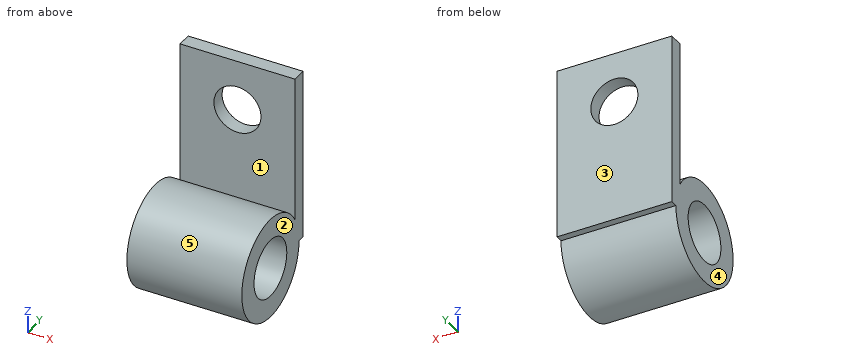
from build123d import *

# Parameters (mm, degrees)
LOOP_SKETCH_R       = 5.575
LOOP_DEPTH          = 6.35
TAB_SKETCH_W        = 18.94
TAB_SKETCH_H        = 1.6
TAB_DEPTH           = 6.35
TUBE_HOLE_SKETCH_R  = 3.195
TUBE_HOLE_DEPTH     = 7.35
MOUNT_HOLE_SKETCH_R = 2.6
MOUNT_HOLE_DEPTH    = 20


with BuildPart() as part:
    # Loop Sketch → Loop (new, symmetric)
    with BuildSketch(Plane(origin=(0, 0, 0), x_dir=(0, 0, -1), z_dir=(1, 0, 0))):
        Circle(LOOP_SKETCH_R)
    extrude(amount=LOOP_DEPTH, both=True)

    # Tab Sketch → Tab (add, symmetric)
    with BuildSketch(Plane(origin=(0, 0, 0), x_dir=(0, 0, -1), z_dir=(1, 0, 0))):
        with Locations((-9.47, 5.575)):
            Rectangle(TAB_SKETCH_W, TAB_SKETCH_H)
    extrude(amount=TAB_DEPTH, both=True)

    # Tube Hole Sketch → Tube Hole (cut, symmetric)
    with BuildSketch(Plane(origin=(0, 0, 0), x_dir=(0, 0, -1), z_dir=(1, 0, 0))):
        Circle(TUBE_HOLE_SKETCH_R)
    extrude(amount=TUBE_HOLE_DEPTH, both=True, mode=Mode.SUBTRACT)

    # Mount Hole Sketch → Mount Hole (cut, symmetric)
    with BuildSketch(Plane(origin=(0, 0, 0), x_dir=(1, 0, 0), z_dir=(0, 1, 0))):
        with Locations(Location((0, -13.44, 0), (0, 0, 270))):
            Circle(MOUNT_HOLE_SKETCH_R)
    extrude(amount=MOUNT_HOLE_DEPTH, both=True, mode=Mode.SUBTRACT)


solid = part.part
Design review of the part built by this model. Coordinates are the model's own, in mm. Face numbers are marked on the shaded views. A direction names the side the tool comes from. Give positions to 0.01 mm unless a question says otherwise; leave off trailing zeros. Order: outer loops, then holes, each group sorted by start corner. A loop starts at its lowest first (then second) coordinate and runs counter-clockwise, first axis right, second up. Notation, with made-up numbers: (-15.75, -39) - (8.25, -39) arc R12 ccw to (8.25, -21) - close; hole circle Ø10 at (-32, 40.5). An arc over 180 degrees is marked (long way). Use CSV: the item, a comma, the result in double quotes. Start each with the question number.
Q1. Take a section at B-B (y = 0). State the section outline as (x, z) points (3 decimals).
Q2. Draft analysis for pull direction Y (two halves, no side actions). For the marked faces 3, 4 and 5, state which applies: pulls with the +Y half, pulls with the -Y half, needs draft (parallel to the pull), parting line crosses it, or undercut.
Q3. Take a section at A-A (x = 0). Count the separate pieces of the cut face and the enclosed holes in it, and give its area (3 significant figures).
Q4. For P1, Ø4, axis at y = 0, z = 0, coming from the +X side; P2, Ø1, axis at x = 2, y = -3.5, coming from the -Z side; P3, Ø0.6, axis at x = 2.5, y = 6, coming from the -Z side; P4, Ø1.5, axis at x = 0, y = 2, coming from the +Z side, all flat-tipped, find the tip position at first contact; note any pin that passes through.
Q5. Machinability: for the marked faces 1 and 2, which of the approach directions +Z, -Z, +X, -X, +Y, -Y give a long, thin tool a straight path to every point of the face, cutting with its end or side? Answer none if there is none.
Q6. Take a section at C-C (z = 13.44). State the section outline as (x, y) points (3 decimals), and give its area (3 significant figures).
Q7. For line 1 (X direction, y = 5.95, z = 13.44); line 2 (Z direction, x = 5.5, y = 5.75); line 3 (Y direction, x = -2, z = -2.5), list the stretches that pass through material, from the lowest coordinate up.
Calculated:
1,outline,"(-6.35, -5.575) - (6.35, -5.575) - (6.35, -3.195) - (-6.35, -3.195) - close; (-6.35, 3.195) - (6.35, 3.195) - (6.35, 5.575) - (-6.35, 5.575) - close"
2,face 3,"pulls with the +Y half"
2,face 4,"needs draft"
2,face 5,"undercut"
3,separate pieces,"2"
3,enclosed holes,"1"
3,area,"86.0 mm²"
4,P1,"passes through"
4,P2,"stops at z = -4.7"
4,P3,"stops at z = 0"
4,P4,"stops at z = 5.43"
5,face 1,"+Z, +X, -X"
5,face 2,"+Z, -Z, +X, +Y, -Y"
6,outline,"(-6.35, 4.775) - (-2.6, 4.775) - (-2.6, 6.375) - (-6.35, 6.375) - close; (2.6, 4.775) - (6.35, 4.775) - (6.35, 6.375) - (2.6, 6.375) - close"
6,area,"12.0 mm²"
7,line 1,"x = -6.35 to -2.6, 2.6 to 6.35"
7,line 2,"z = 0 to 18.94"
7,line 3,"y = -4.98 to -1.99, 1.99 to 4.98"
